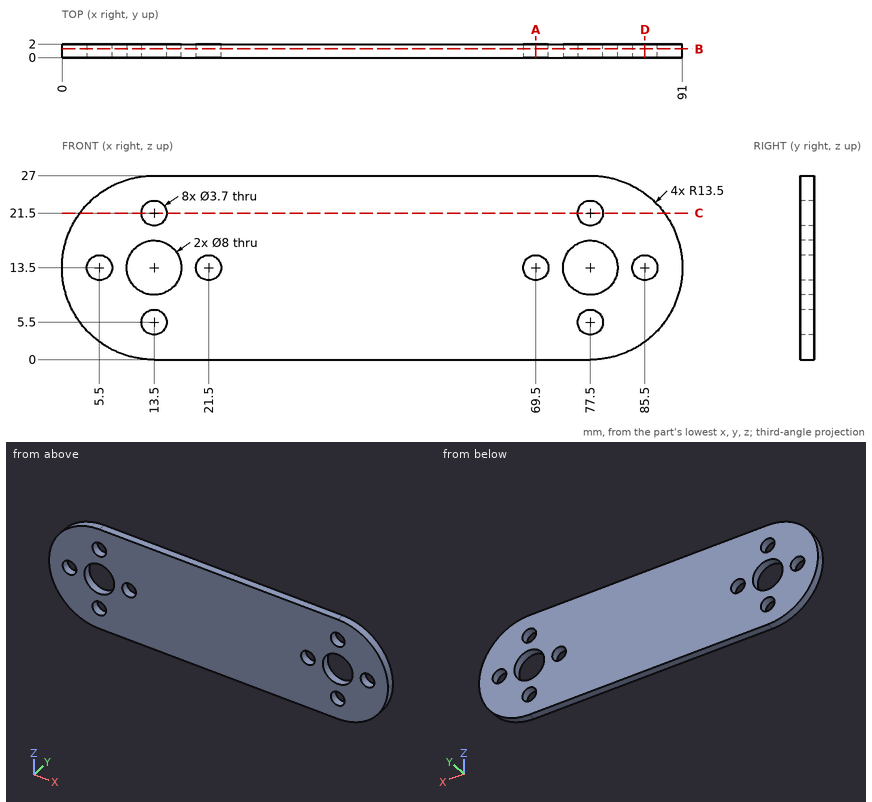
Here's the drawing with two shaded views (mm, measured from the low corner). I have some questions. Round coordinates to 2 decimals unless told otherwise and drop trailing zeros. Loops run counter-clockwise (first coordinate to the right, second up) from the corner with the lowest first, then second, coordinate; pieces in that order, holes last. Notation, with made-up numbers: M 3,24.5 L 8,24.5 A21 cw 8,39.5 Z; hole C -24.75,52 d2. An arc over 180 degrees is marked long. Put each result on its own line as item: value.
Q1. Imagine slicing it at C-C (z = 21.5). Write out the boundary of the cut face in (x, y).
Check result:
outline: M 2.63,0 L 11.65,0 L 11.65,2 L 2.63,2 Z; M 15.35,0 L 75.65,0 L 75.65,2 L 15.35,2 Z; M 79.35,0 L 88.37,0 L 88.37,2 L 79.35,2 Z
Q2. For pin 1 (1 mm diameter, centred on y = 1.5, z = 9.5, fed in from +X), with a flat end and sliding along its axis, tell me the tip position at first contact or that it passes through.
Check result:
pin 1: x = 90.54
Q3. I need wall thicknesses on probe 1 along Z at (x, y) = (13.5, 0.8); probe 2 along X at (y, z) = (1.5, 11); probe 3 along Z at (x, y) = (21.5, 1.15). Which ranges of each line are inside material? Lowest first, please.
Check result:
probe 1: 0 to 3.65, 7.35 to 9.5, 17.5 to 19.65, 23.35 to 27
probe 2: 0.23 to 10.38, 16.62 to 74.38, 80.62 to 90.77
probe 3: 0 to 11.65, 15.35 to 27
Q4. Imagine slicing it at A-A (x = 69.5). Write out the boundary of the cut face in (y, z).
Check result:
outline: M 0,0 L 2,0 L 2,11.65 L 0,11.65 Z; M 0,15.35 L 2,15.35 L 2,27 L 0,27 Z
Q5. Imagine slicing it at B-B (y = 1.3). State how many separate pieces and enclosed holes the cut face has, then the cut area to 3 significant figures.
Check result:
separate pieces: 1
enclosed holes: 10
area: 2,110 mm2
Q6. Imagine slicing it at D-D (x = 85.5). Write out the boundary of the cut face in (y, z), then the cut area to 3 significant figures.
Check result:
outline: M 0,2.63 L 2,2.63 L 2,11.65 L 0,11.65 Z; M 0,15.35 L 2,15.35 L 2,24.37 L 0,24.37 Z
area: 36.1 mm2
